from build123d import *

# Parameters (mm, degrees)
THICKEN1_T1 = 2


with BuildPart() as body_1:
    # Sketch1 → Surface-Plane1: a flat surface bounded by the sketch
    with BuildSketch(Plane(origin=(0, 0, 0), x_dir=(0, 0, -1), z_dir=(1, 0, 0)), mode=Mode.PRIVATE) as surface_plane1_1_region:
        with BuildLine():
            Line((0, 642), (-40, 642))
            ThreePointArc((-40, 642), (-66, 635.033320997), (-85.033320997, 616))
            Line((-85.033320997, 616), (-401.033320997, 68.671944808))
            ThreePointArc((-401.033320997, 68.671944808), (-403.165451776, 57.95299954), (-398.331704413, 48.151129528))
            Line((-398.331704413, 48.151129528), (-348.766361322, -1.414213562))
            Line((-348.766361322, -1.414213562), (0, 0))
            Line((0, 0), (0, 642))
        make_face()
    surface_plane1_1 = surface_plane1_1_region.sketch.faces()[0]
    add(Solid.thicken(surface_plane1_1, THICKEN1_T1))


solid = body_1.part
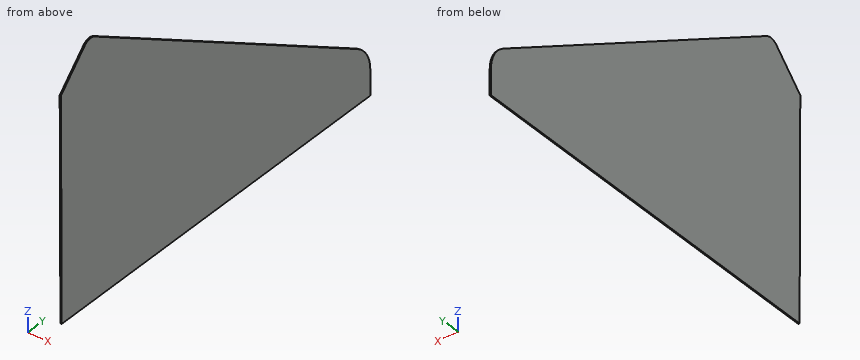
Verification items for the finished model (mm, model axes). Give positions to 0.01 mm unless a question says otherwise; leave off trailing zeros. Loops run counter-clockwise (first coordinate to the right, second up) from the corner with the lowest first, then second, coordinate; pieces in that order, holes last.
1. Cross-section at A-A on x = 0.7. Record the cut outline in (y, z), and give its area (3 significant figures).
Derived:
outline: (-1.41, 348.77) - (0, 0) - (642, 0) - (642, 40) arc R52 ccw to (616, 85.03) - (68.67, 401.03) arc R17 ccw to (48.15, 398.33) - close
area: 161,000 mm2
2. Cross-section at C-C on y = 223.5. Record the cut outline in (x, z), and give its area (3 significant figures).
Derived:
outline: (0, 0) - (2, 0) - (2, 311.64) - (0, 311.64) - close
area: 623 mm2
3. Cross-section at B-B on z = 276.5. Record the cut outline in (x, y).
Derived:
outline: (0, -1.12) - (2, -1.12) - (2, 284.37) - (0, 284.37) - close
4. Material ranges on probe 1 along Y at (x, z) = (1.05, 258.5); probe 2 along Y at (x, z) = (0.95, 62.5); probe 3 along Z at (x, y) = (0.6, 241), recorded low to high.
Derived:
probe 1: y = -1.05 to 315.55
probe 2: y = -0.25 to 636.88
probe 3: z = 0 to 301.54
5. Go/stop test with a flat-tipped pin: P1, Ø1, axis at x = 0.5, y = 430, coming from the +Z side. Record where the tip stops, or that it passes through.
Derived:
P1: stops at z = 192.71
